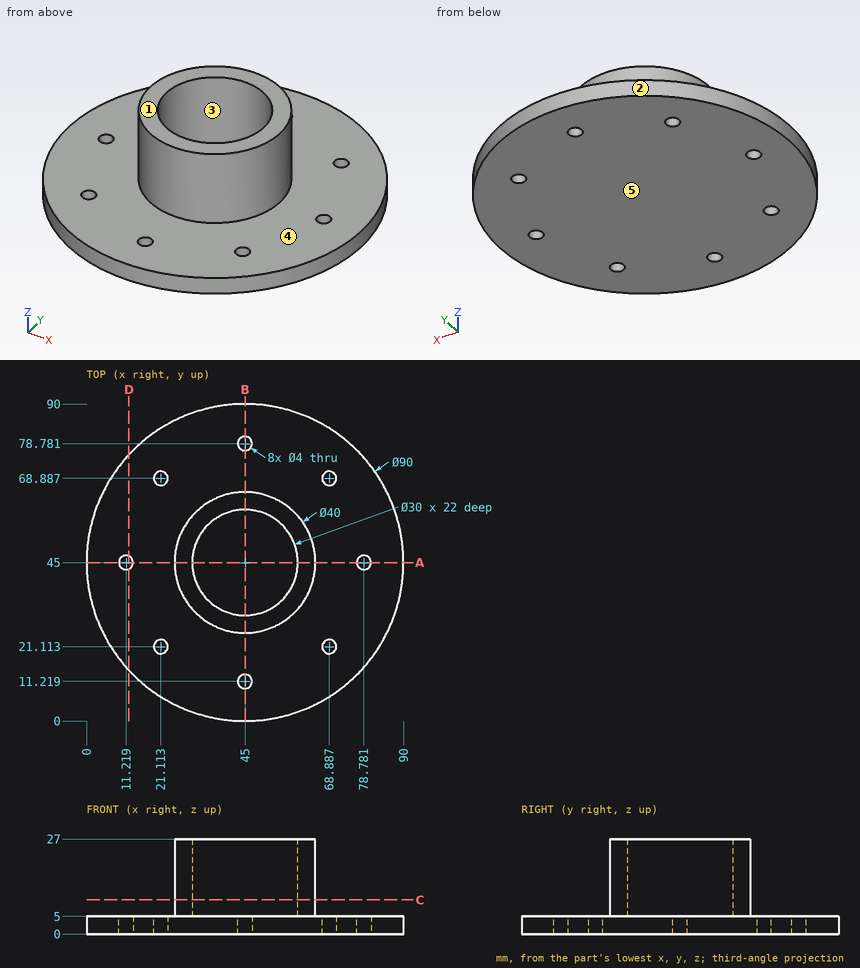
Study the drawing (mm; zero at the part's minimum x, y, z) and answer. A direction names the side the tool comes from. Round coordinates to 2 decimals unless told otherwise and drop trailing zeros. Write each loop counter-clockwise with the first axis right and the second up, starting at its lowest first coordinate (ties: lowest second). Pieces come first, ordered by that corner, then holes.
1) Which of the six approach directions +Z, -Z, +X, -X, +Y, -Y give full straight-line access (tool end or side, diameter ignored) to the marked faces 4 and 5?
2) A cutting plane is placed at A-A on y = 45. Determine the outline of the cut face in (x, z).
3) Flat-ended cylindrical pins translate along their axes: P1, Ø3.5, axis at x = 45, y = 11.22, coming from the -Z side; P2, Ø18, axis at x = 45, y = 45, coming from the +Z side; P3, Ø6, axis at y = 42.5, z = 8.5, coming from the +X side; P4, Ø12, axis at x = 30.5, z = 10.5, coming from the +Y side. Find the tip coordinate at first contact, or state that the pin passes through.
4) Consider probe 1 along Y at (x, z) = (45, 3.25); probe 2 along Z at (x, y) = (14.5, 57); probe 3 along X at (y, z) = (54.5, 19.5). Determine where each line is inside the solid, lowest interval first.
5) A cutting plane is placed at C-C on z = 9.75. Determine the outline of the cut face in (x, y), and give its area (3 significant figures).
6) Determine the mould class of the marked faces 1, 2 and 3 for opening direction Y: pulls with the +Y half, pulls with the -Y half, needs draft (parallel to the pull), parting line crosses it, or undercut.
7) A cutting plane is placed at D-D on x = 12. Determine the outline of the cut face in (y, z).
Entries:
1. face 4: +Z
1. face 5: -Z, +X, -X, +Y, -Y
2. outline: (0, 0) - (9.22, 0) - (9.22, 5) - (0, 5) - close; (13.22, 0) - (76.78, 0) - (76.78, 5) - (65, 5) - (65, 27) - (60, 27) - (60, 5) - (30, 5) - (30, 27) - (25, 27) - (25, 5) - (13.22, 5) - close; (80.78, 0) - (90, 0) - (90, 5) - (80.78, 5) - close
3. P1: passes through
3. P2: stops at z = 5
3. P3: stops at x = 65
3. P4: stops at y = 88.34
4. probe 1: y = 0 to 9.22, 13.22 to 76.78, 80.78 to 90
4. probe 2: z = 0 to 5
4. probe 3: x = 27.4 to 33.39, 56.61 to 62.6
5. outline: circle Ø40 at (45, 45); hole circle Ø30 at (45, 45)
5. area: 550 mm2
6. face 1: needs draft
6. face 2: parting line crosses it
6. face 3: undercut
7. outline: (14.41, 0) - (43.16, 0) - (43.16, 5) - (14.41, 5) - close; (46.84, 0) - (75.59, 0) - (75.59, 5) - (46.84, 5) - close
